```python
from build123d import *

# Parameters (mm, degrees)
SKETCH1_R           = 1.5
BOSS_EXTRUDE1_DEPTH = 2


with BuildPart() as part:
    # Sketch1 → Boss-Extrude1 (new body)
    with BuildSketch(Plane.XY):
        with BuildLine():
            Line((19.021561934, 0), (40.542646089, 4.662222335))
            ThreePointArc((40.542646089, 4.662222335), (45.821499943, 11.972802233), (39.114495851, 17.999988357))
            Line((39.114495851, 17.999988357), (19.021561934, 17.999988357))
            Line((19.021561934, 17.999988357), (19.021561934, 13.999988357))
            Line((19.021561934, 13.999988357), (17, 13.999988357))
            Line((17, 13.999988357), (17, 17.999988357))
            Line((17, 17.999988357), (13, 17.999988357))
            Line((13, 17.999988357), (13, 13.999988357))
            Line((13, 13.999988357), (9, 13.999988357))
            Line((9, 13.999988357), (9, 17.999988357))
            Line((9, 17.999988357), (5, 17.999988357))
            Line((5, 17.999988357), (5, 13.999988357))
            Line((5, 13.999988357), (0, 13.999988357))
            Line((0, 13.999988357), (0, 4))
            Line((0, 4), (5, 4))
            Line((5, 4), (5, 0))
            Line((5, 0), (9, 0))
            Line((9, 0), (9, 4))
            Line((9, 4), (13, 4))
            Line((13, 4), (13, 0))
            Line((13, 0), (17, 0))
            Line((17, 0), (17, 4))
            Line((17, 4), (19.021561934, 4))
            Line((19.021561934, 4), (19.021561934, 0))
        make_face()
        with Locations((39.114495851, 11.254645274)):
            Circle(SKETCH1_R, mode=Mode.SUBTRACT)
        with Locations((3.920490093, 8.999988357)):
            Circle(SKETCH1_R, mode=Mode.SUBTRACT)
    extrude(amount=BOSS_EXTRUDE1_DEPTH)


solid = part.part
```
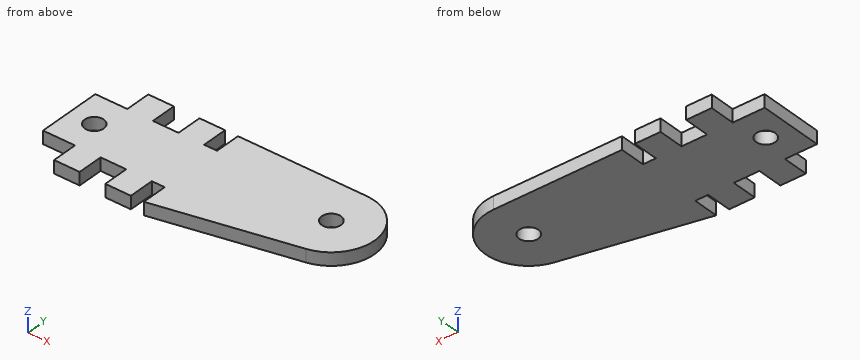
The model under review builds one solid part; all positions refer to its coordinate system, in mm. Give positions to 0.01 mm unless a question says otherwise; leave off trailing zeros. Write each loop counter-clockwise with the first axis right and the second up, starting at its lowest first coordinate (ties: lowest second). Pieces come first, ordered by that corner, then holes. Notation, with made-up numbers: M 85,67 L 104,67 A16 ccw 104,71 Z; hole C 40.25,6 d3. An arc over 180 degrees is marked long. Answer in a Markdown table with one row per item.
Item 1: For line 1 along X through (y, z) = (9.5, 0.95); line 2 along Y through (x, z) = (40, 0.75); line 3 along X through (y, z) = (8.5, 0.8), list the stretches that pass through material, from the lowest coordinate up.
Check sheet entries:
| item | result |
|---|---|
| line 1 | 0 to 2.51, 5.33 to 45.63 |
| line 2 | 4.54 to 10.04, 12.47 to 17.94 |
| line 3 | 0 to 2.51, 5.33 to 45.27 |
Item 2: Add section C-C on y = 12.25. Give the boundary of the cut face in (x, z), plus the area to 3 significant figures.
Check sheet entries:
| item | result |
|---|---|
| outline | M 0,0 L 37.99,0 L 37.99,2 L 0,2 Z; M 40.24,0 L 45.79,0 L 45.79,2 L 40.24,2 Z |
| area | 87.1 mm2 |
Item 3: Add section D-D on z = 0.45. Give the boundary of the cut face in (x, y), plus the area to 3 significant figures.
Check sheet entries:
| item | result |
|---|---|
| outline | M 0,4 L 5,4 L 5,0 L 9,0 L 9,4 L 13,4 L 13,0 L 17,0 L 17,4 L 19.02,4 L 19.02,0 L 40.54,4.66 A6.75 ccw 39.11,18 L 19.02,18 L 19.02,14 L 17,14 L 17,18 L 13,18 L 13,14 L 9,14 L 9,18 L 5,18 L 5,14 L 0,14 Z; hole C 3.92,9 d3; hole C 39.11,11.25 d3 |
| area | 630 mm2 |
Item 4: For P1, Ø1, axis at x = 11.5, z = 1, coming from the +Y side; P2, Ø1, axis at y = 1, z = 1.5, coming from the -X side; P3, Ø1, axis at y = 5, z = 1, coming from the +X side; P4, Ø2.5, axis at x = 39.11, y = 11.25, coming from the -Z side, all flat-tipped, find the tip position at first contact; note any pin that passes through.
Check sheet entries:
| item | result |
|---|---|
| P1 | y = 14 |
| P2 | x = 5 |
| P3 | x = 42.63 |
| P4 | through |
Item 5: Add section A-A on y = 16.75. Give the boundary of the cut face in (x, z).
Check sheet entries:
| item | result |
|---|---|
| outline | M 5,0 L 9,0 L 9,2 L 5,2 Z; M 13,0 L 17,0 L 17,2 L 13,2 Z; M 19.02,0 L 43.03,0 L 43.03,2 L 19.02,2 Z |
Item 6: Add section B-B on x = 40. Give the boundary of the cut face in (y, z).
Check sheet entries:
| item | result |
|---|---|
| outline | M 4.54,0 L 10.04,0 L 10.04,2 L 4.54,2 Z; M 12.47,0 L 17.94,0 L 17.94,2 L 12.47,2 Z |
